Answer from the drawing. Dimensions are ordinates in mm from the lowest x, y and z of the part. Give positions to 0.01 mm unless a question says otherwise; leave off trailing zeros. Loops run counter-clockwise (first coordinate to the right, second up) from the corner with the lowest first, then second, coordinate; pieces in that order, holes last.
(1) Each of these flat-tipped pins is pushed along its axis until it touches: P1, Ø1, axis at y = 4, z = 11.5, coming from the -X side; P2, Ø3, axis at x = 11.5, y = 1.5, coming from the +Z side (1 decimal); P3, Ø2, axis at x = 30, y = 1, coming from the -Z side. Where does it stop, or does it pass through?
(2) Find section D-D, the plane z = 14. Write down the section's boundary in (x, y).
(3) Find section A-A, the plane z = 78. Write down the section's boundary in (x, y), then the cut area to 3 significant figures.
(4) Find section C-C, the plane x = 11. Write down the section's boundary in (y, z) (1 decimal).
(5) Find section B-B, the plane y = 2. State how many separate pieces and enclosed holes the cut face has, then the cut area to 3 significant figures.
(6) Straight lines are drawn through the part: probe 1 along X at (y, z) = (4.4, 74); probe 2 along Z at (x, y) = (7.5, 2.2) (1 decimal); probe 3 along X at (y, z) = (4, 82.5). For each, find the intervals that lie inside material, in ascending order.
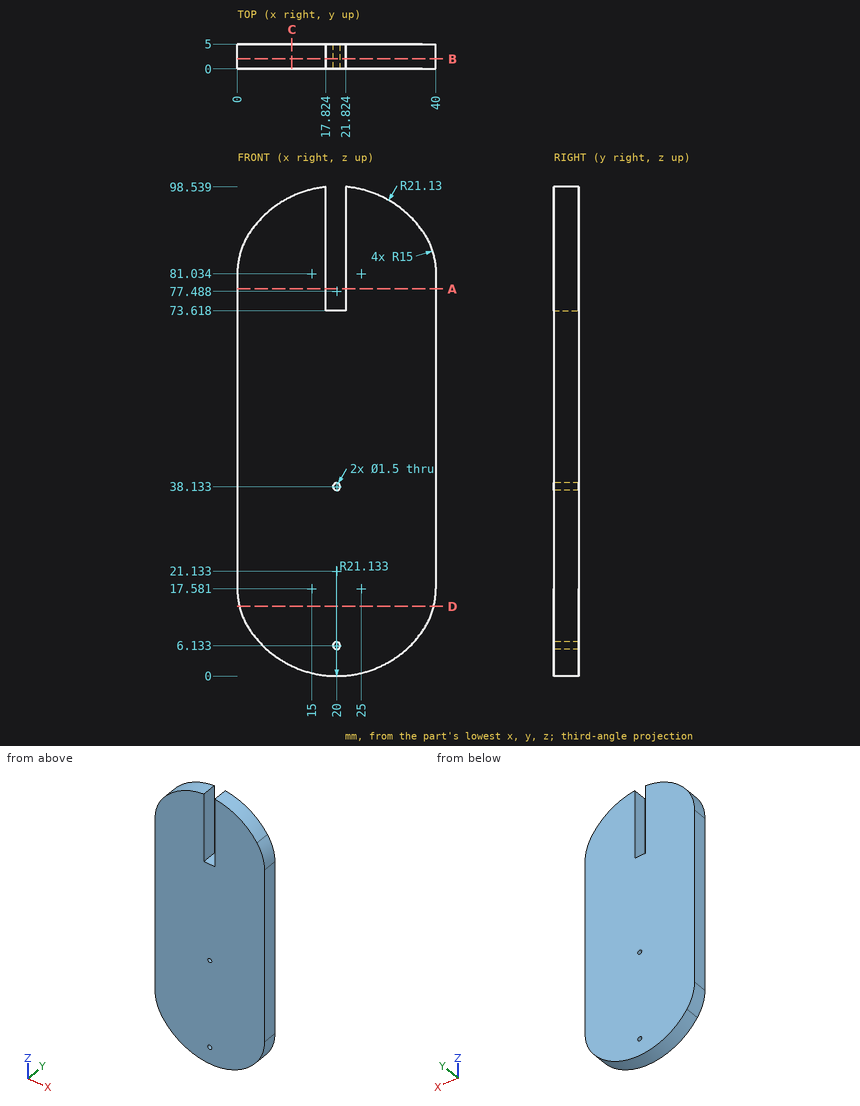
Entries:
1. P1: stops at x = 1.08
1. P2: stops at z = 97.4
1. P3: stops at z = 2.01
2. outline: (0.43, 0) - (39.57, 0) - (39.57, 5) - (0.43, 5) - close
3. outline: (0, 0) - (17.82, 0) - (17.82, 5) - (0, 5) - close; (21.82, 0) - (40, 0) - (40, 5) - (21.82, 5) - close
3. area: 180 mm2
4. outline: (0, 2) - (5, 2) - (5, 96.6) - (0, 96.6) - close
5. separate pieces: 1
5. enclosed holes: 2
5. area: 3,530 mm2
6. probe 1: x = 0 to 17.82, 21.82 to 40
6. probe 2: z = 4.1 to 94.5
6. probe 3: x = 0.07 to 17.82, 21.82 to 39.93
